Design review of the part shown in the three views and the two pictorial views. Dimensions are in mm from the part's minimum x, y and z. A direction names the side the tool comes from. Give positions to 0.01 mm unless a question says otherwise; leave off trailing zeros. Order: outer loops, then holes, each group sorted by start corner. A loop starts at its lowest first (then second) coordinate and runs counter-clockwise, first axis right, second up. Notation, with made-up numbers: M -9,29.25 L -4,29.25 A22 ccw -4,64.25 Z; hole C 55,-16 d1. An arc over 180 degrees is marked long. Answer as a JSON object with one key per item and string values.
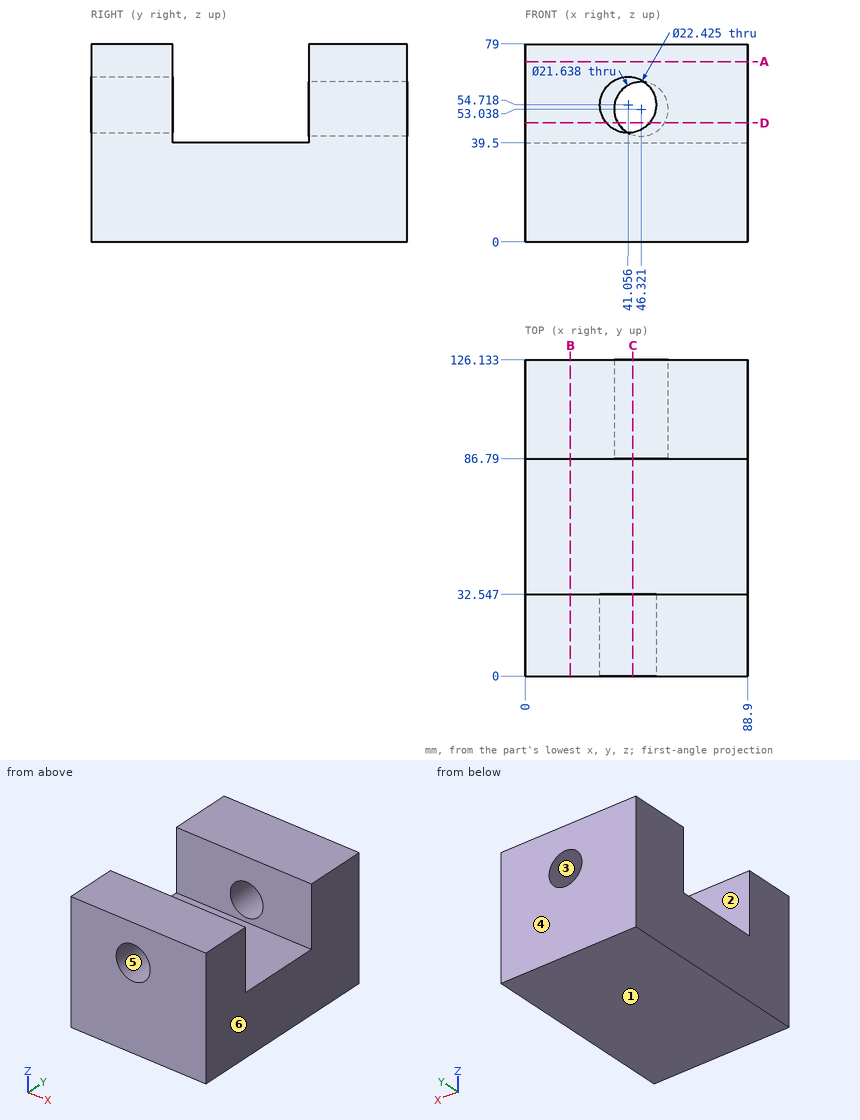
(1) We need section C-C (x = 43). Write out the cut boundary in (y, z) (1 decimal).
Checked values:
{"outline": "M 0,0 L 126.1,0 L 126.1,42.7 L 86.8,42.7 L 86.8,39.5 L 32.5,39.5 L 32.5,43.7 L 0,43.7 Z; M 0,65.8 L 32.5,65.8 L 32.5,79 L 0,79 Z; M 86.8,63.3 L 126.1,63.3 L 126.1,79 L 86.8,79 Z"}
(2) We need section D-D (z = 47.5). Write out the cut boundary in (x, y) (1 decimal), plus the area to 3 significant figures.
Checked values:
{"outline": "M 0,0 L 32.5,0 L 32.5,32.5 L 0,32.5 Z; M 0,86.8 L 37,86.8 L 37,126.1 L 0,126.1 Z; M 49.6,0 L 88.9,0 L 88.9,32.5 L 49.6,32.5 Z; M 55.6,86.8 L 88.9,86.8 L 88.9,126.1 L 55.6,126.1 Z", "area": "5,100 mm^2"}
(3) To check wall thickness, follow L1, parallel to Y at x = 43, z = 71; L2, parallel to X at y = 23.5, z = 51.5 (1 decimal); L3, parallel to Z at x = 49, y = 17.5 (1 decimal). State the ranges of each line that lie inside material, in increasing order. Write a range as from..to.
Checked values:
{"L1": "y = 0..32.55, 86.79..126.13", "L2": "x = 0..30.3, 51.8..88.9", "L3": "z = 0..46.8, 62.6..79"}
(4) Insertion check: pin 1 (1 mm diameter, centred on x = 14.5, z = 25, fed in from -Y); pin 2 (19.5 mm diameter, centred on x = 46.32, z = 53.04, fed in from +Y). Each pin has a flat end and moves straight along its axis. Give the tip position at first contact, or say it passes through.
Checked values:
{"pin 1": "stops at y = 0", "pin 2": "stops at y = 32.55"}
(5) We need section A-A (z = 72). Write out the cut boundary in (x, y).
Checked values:
{"outline": "M 0,0 L 88.9,0 L 88.9,32.55 L 0,32.55 Z; M 0,86.79 L 88.9,86.79 L 88.9,126.13 L 0,126.13 Z"}
(6) We need section B-B (x = 18). Write out the cut boundary in (y, z).
Checked values:
{"outline": "M 0,0 L 126.13,0 L 126.13,79 L 86.79,79 L 86.79,39.5 L 32.55,39.5 L 32.55,79 L 0,79 Z"}
(7) Draft analysis for pull direction X (two halves, no side actions). For the marked faces 3, 4, 5 and 6, state which applies: +X half, -X half, draft (parallel to the pull), parting line (faces both ways), or undercut.
Checked values:
{"face 3": "undercut", "face 4": "draft", "face 5": "undercut", "face 6": "+X half"}
(8) Tool access review of the marked faces 1 and 2: name each direction out of +Z, -Z, +X, -X, +Y, -Y from which nothing blocks a thin tool from reaching the whole face with its end or side.
Checked values:
{"face 1": "-Z, +X, -X, +Y, -Y", "face 2": "+Z, +X, -X"}
